from build123d import *

# Parameters (mm, degrees)
F0_W      = 279.4
F0_H      = 381
F1_DEPTH  = 1.98374
F6_R      = 12.0015
F6_R_2    = 1.5875
F3_R      = 30.1625
F3_R_2    = 2.54
F5_W      = 71.12
F5_H      = 45.339
F5_R      = 2.54
F7_R      = 12.0015
F7_R_2    = 1.5875
F7_R_3    = 6.35
F4_W      = 22.225
F4_H      = 28.1178
F8_W      = 66.675
F8_H      = 32.512
F8_R      = 2.54
F9_DEPTH  = 25.4
F11_DEPTH = 25.4
F12_R     = 2.54
F13_DEPTH = 25.4
F14_R     = 6.35


with BuildPart() as f1:
    # F0 (on Front) → F1 (new body)
    with BuildSketch(Plane.XZ):
        Rectangle(F0_W, F0_H)
    extrude(amount=F1_DEPTH)

    # F6 (on face) + F3 (on face) + F5 (on face) + F7 (on face) + F4 (on face) + F8 (on face) → F9 (cut)
    with BuildSketch(Plane.XZ.offset(1.98374)):
        with Locations((-79.375, -57.15)):
            Circle(F6_R)
        with Locations((-88.8365, -45.1485)):
            Circle(F6_R_2)
        with Locations((-69.9135, -69.1515)):
            Circle(F6_R_2)
        with Locations((-47.625, -57.15)):
            Circle(F6_R)
        with Locations((-57.0865, -45.1485)):
            Circle(F6_R_2)
        with Locations((-38.1635, -69.1515)):
            Circle(F6_R_2)
        with Locations((-15.875, -57.15)):
            Circle(F6_R)
        with Locations((-25.3365, -45.1485)):
            Circle(F6_R_2)
        with Locations((-6.4135, -69.1515)):
            Circle(F6_R_2)
        with Locations((15.875, -57.15)):
            Circle(F6_R)
        with Locations((6.4135, -45.1485)):
            Circle(F6_R_2)
        with Locations((25.3365, -69.1515)):
            Circle(F6_R_2)
        with Locations((47.625, -57.15)):
            Circle(F6_R)
        with Locations((38.1635, -45.1485)):
            Circle(F6_R_2)
        with Locations((57.0865, -69.1515)):
            Circle(F6_R_2)
        with Locations((79.375, -57.15)):
            Circle(F6_R)
        with Locations((69.9135, -45.1485)):
            Circle(F6_R_2)
        with Locations((88.8365, -69.1515)):
            Circle(F6_R_2)
    with BuildSketch(Plane.XZ.offset(1.98374)):
        with Locations((-76.2, 12.7)):
            Circle(F3_R)
        with Locations((-76.2, 47.1551)):
            Circle(F3_R_2)
        with Locations((-41.7449, 12.7)):
            Circle(F3_R_2)
        with Locations((-76.2, -21.7551)):
            Circle(F3_R_2)
        with Locations((-110.6551, 12.7)):
            Circle(F3_R_2)
    with BuildSketch(Plane.XZ.offset(1.98374)):
        with Locations((-48.26, 107.95)):
            Rectangle(F5_W, F5_H)
        with Locations((48.26, 107.95)):
            Rectangle(F5_W, F5_H)
        with Locations((-96.52, 107.95)):
            Circle(F5_R)
        with Locations((96.52, 107.95)):
            Circle(F5_R)
        with Locations((0, 107.95)):
            Circle(F5_R)
    with BuildSketch(Plane.XZ.offset(1.98374)):
        with Locations((-47.625, -95.25)):
            Circle(F7_R)
        with Locations((-57.0865, -83.2485)):
            Circle(F7_R_2)
        with Locations((-38.1635, -107.2515)):
            Circle(F7_R_2)
        with Locations((-15.875, -95.25)):
            Circle(F7_R)
        with Locations((-25.3365, -83.2485)):
            Circle(F7_R_2)
        with Locations((-6.4135, -107.2515)):
            Circle(F7_R_2)
        with Locations((15.875, -95.25)):
            Circle(F7_R)
        with Locations((6.4135, -83.2485)):
            Circle(F7_R_2)
        with Locations((25.3365, -107.2515)):
            Circle(F7_R_2)
        with Locations((47.625, -95.25)):
            Circle(F7_R)
        with Locations((38.1635, -83.2485)):
            Circle(F7_R_2)
        with Locations((57.0865, -107.2515)):
            Circle(F7_R_2)
        with Locations((-79.375, -95.25)):
            Circle(F7_R_3)
        with Locations((79.375, -95.25)):
            Circle(F7_R_3)
    with BuildSketch(Plane.XZ.offset(1.98374)):
        with Locations((0, 12.7)):
            Rectangle(F4_W, F4_H)
    with BuildSketch(Plane.XZ.offset(1.98374)):
        with Locations((0, -139.7)):
            Rectangle(F8_W, F8_H)
        with Locations((-41.8465, -139.7)):
            Circle(F8_R)
        with Locations((41.8465, -139.7)):
            Circle(F8_R)
    extrude(amount=-F9_DEPTH, mode=Mode.SUBTRACT)

    # F10 (on face) → F11 (cut)
    with BuildSketch(Plane.XZ.offset(1.98374)):
        with BuildLine():
            Line((139.7, 71.3907683632), (81.7796158184, 13.4703841816))
            ThreePointArc((81.7796158184, 13.4703841816), (76.2, 0), (81.7796158184, -13.4703841816))
            Line((81.7796158184, -13.4703841816), (139.7, -71.3907683632))
            Line((139.7, -71.3907683632), (139.7, 71.3907683632))
        make_face()
    extrude(amount=-F11_DEPTH, mode=Mode.SUBTRACT)

    # F12 (on face) → F13 (cut)
    with BuildSketch(Plane.XZ.offset(1.98374)):
        with Locations((-133.35, 184.15)):
            Circle(F12_R)
        with Locations((133.35, 184.15)):
            Circle(F12_R)
        with Locations((133.35, 92.075)):
            Circle(F12_R)
        with Locations((133.35, -92.075)):
            Circle(F12_R)
        with Locations((133.35, -184.15)):
            Circle(F12_R)
        with Locations((-133.35, -184.15)):
            Circle(F12_R)
        with Locations((-133.35, -92.075)):
            Circle(F12_R)
        with Locations((-133.35, 92.075)):
            Circle(F12_R)
        with Locations((-133.35, 0)):
            Circle(F12_R)
        with Locations((-44.45, 184.15)):
            Circle(F12_R)
        with Locations((-44.45, -184.15)):
            Circle(F12_R)
        with Locations((44.45, 184.15)):
            Circle(F12_R)
        with Locations((44.45, -184.15)):
            Circle(F12_R)
        with Locations((69.85, 0)):
            Circle(F12_R)
    extrude(amount=-F13_DEPTH, mode=Mode.SUBTRACT)

    # F14
    f14_edges = [f1.edges().sort_by_distance(p)[0] for p in [
        (-139.7, -0.99187, 190.5),
        (139.7, -0.99187, 190.5),
        (139.7, -0.99187, 71.390768),
        (139.7, -0.99187, -71.390768),
        (139.7, -0.99187, -190.5),
        (-139.7, -0.99187, -190.5),
    ]]
    fillet(f14_edges, radius=F14_R)


solid = f1.part
Can you work these out from the model? Positions are in its coordinate system, mm. A direction names the side the tool comes from. Round coordinates to 2 decimals unless told otherwise and drop trailing zeros. Loops run counter-clockwise (first coordinate to the right, second up) from the corner with the lowest first, then second, coordinate; pieces in that order, holes last. Notation, with made-up numbers: (26.5, 58.5) - (55.5, 58.5) arc R19 cw to (55.5, 91.5) - close; hole circle Ø11 at (39, 79.5). An arc over 180 degrees is marked (long way). Write item = value, one per line. Start each with the question number.
(1) For faces 3 (the face through (110.2, -1.01, 41.89)), 4 (the face through (53.16, -1.01, -105.9)), which set-ups out of +Z, -Z, +X, -X, +Y, -Y let a thin tool reach every point of the face, with its end or its side?
(2) If we mould it in two halves opening along Z, with no side actions, what happens to faces 1 (the face through (-42.09, -1.01, -105.9)), 2 (the face through (-33, 0, 3))? For each: released by +Z, released by -Z, zero draft, split by the parting line, or undercut.
(3) If we section it at C-C (y = -1.15): Give the number of separate pieces and of enclosed holes in the cut face, and give its area (3 significant figures).
(4) If we section it at A-A (z = -130.5): Please give me the cut outline in (x, y).
(5) If we section it at B-B (z = -9): Please give me the cut outline in (x, y).
(6) For P1, Ø4, axis at x = 44.45, z = 184.15, coming from the -Y side, with a flat end and sliding along its axis, tell me the tip position at first contact or that it passes through.
(7) If I drill on probe 1 along X at (y, z) = (-1.4, -184.15); probe 2 along Z at (x, y) = (-133.35, -1.5) (3 decimals); probe 3 along Z at (x, y) = (44.45, -0.6), over which ranges is the centre line in solid material (lowest first)? Write a range as [from, to].
Ans:
q1.face_3 = +X, +Y, -Y
q1.face_4 = +Y, -Y
q2.face_1 = undercut
q2.face_2 = zero draft
q3.separate_pieces = 1
q3.enclosed_holes = 60
q3.area = 83,900 mm²
q4.outline = (-139.7, -1.98) - (-33.34, -1.98) - (-33.34, 0) - (-139.7, 0) - close; (33.34, -1.98) - (139.7, -1.98) - (139.7, 0) - (33.34, 0) - close
q5.outline = (-139.7, -1.98) - (-97.15, -1.98) - (-97.15, 0) - (-139.7, 0) - close; (-55.25, -1.98) - (78.46, -1.98) - (78.46, 0) - (-55.25, 0) - close
q6.P1 = through
q7.probe_1 = [-139.7, -135.89], [-130.81, -46.99], [-41.91, 41.91], [46.99, 130.81], [135.89, 139.7]
q7.probe_2 = [-190.5, -186.69], [-181.61, -94.615], [-89.535, -2.54], [2.54, 89.535], [94.615, 181.61], [186.69, 190.5]
q7.probe_3 = [-190.5, -186.69], [-181.61, -106.82], [-83.68, -68.72], [-45.58, 85.28], [130.62, 181.61], [186.69, 190.5]
